Part model, mm, in its own coordinate system. Face numbers are marked on the shaded views. Give positions to 0.01 mm unless a question says otherwise; leave off trailing zeros. Loops run counter-clockwise (first coordinate to the right, second up) from the corner with the lowest first, then second, coordinate; pieces in that order, holes last. Notation, with made-up numbers: (84, -17) -> (102, -17) arc R28 cw to (102, 18) -> close; hole circle Ø9 at (-31, 85). An arc over 180 degrees is marked (long way). One line per question, with ' | ' between items.
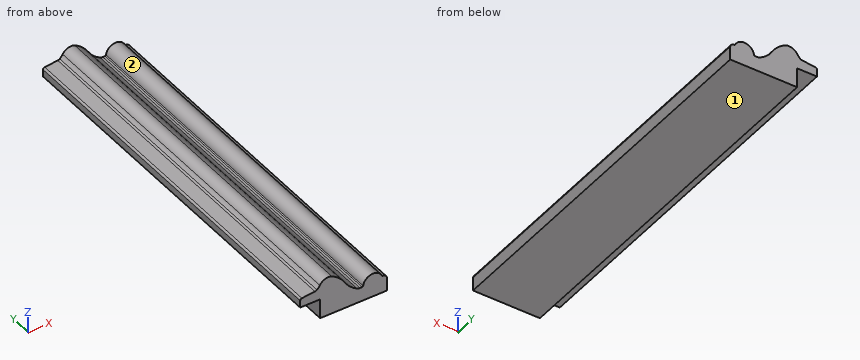
```python
from build123d import *

# Parameters (mm, degrees)
F1_DEPTH = 152.4


# Not quite as in the source:
# - ends of sketch curves that miss each other by under 0.0002 mm in the source are joined


with BuildPart() as f1:
    # F0 (on Front) → F1 (new body)
    with BuildSketch(Plane.XZ):
        with BuildLine():
            Line((-9.4615, 0.028575), (-9.4615, -7.908925))
            Line((-9.4615, -7.908925), (17.4625, -7.908925))
            Line((17.4625, -7.908925), (17.4625, -2.65938))
            ThreePointArc((17.4625, -2.65938), (16.9760741715, -1.5035311682), (15.8095437434, -1.0433101682))
            ThreePointArc((15.8095437434, -1.0433101682), (15.5930919547, -0.9817228233), (15.4491526844, -0.8087322213))
            ThreePointArc((15.4491526844, -0.8087322213), (11.2653307166, 1.5970590296), (7.8607199392, -1.8235935338))
            ThreePointArc((7.8607199392, -1.8235935338), (7.736905149, -2.0587727487), (7.4894692803, -2.1557927219))
            Line((7.4894692803, -2.1557927219), (7.4829161901, -2.1558009151))
            Line((7.4829161901, -2.1558009151), (6.603492, -2.1559774))
            ThreePointArc((6.603492, -2.1559774), (5.9901232061, -2.0809037525), (5.413035163, -1.8599360759))
            ThreePointArc((5.413035163, -1.8599360759), (2.7666336142, 0.0131384296), (0.682874392, 2.4970459891))
            ThreePointArc((0.682874392, 2.4970459891), (-1.6202189431, 5.441919304), (-4.6831053409, 7.585571483))
            ThreePointArc((-4.6831053409, 7.585571483), (-7.435761648, 7.7094554069), (-9.5520790293, 5.9448968563))
            ThreePointArc((-9.5520790293, 5.9448968563), (-10.089729001, 5.2101835463), (-10.7216915696, 4.5548251488))
            ThreePointArc((-10.7216915696, 4.5548251488), (-11.0931160448, 4.3208677831), (-11.52199893, 4.2273251642))
            ThreePointArc((-11.52199893, 4.2273251642), (-14.1558174385, 3.9550500254), (-16.7874935974, 3.6627947922))
            ThreePointArc((-16.7874935974, 3.6627947922), (-17.2692415305, 3.4129116875), (-17.4625, 2.9057854))
            Line((-17.4625, 2.9057854), (-17.4625, 0.028575))
            Line((-17.4625, 0.028575), (-9.4615, 0.028575))
        make_face()
    extrude(amount=F1_DEPTH)


solid = f1.part
```
1) Pin check, flat tips, straight feed: P1, Ø0.7, axis at x = 7, y = -104.5, coming from the +Z side; P2, Ø4, axis at x = 9.5, y = -16.5, coming from the +Z side; P3, Ø6.5, axis at x = -14.5, y = -89, coming from the -Z side. Stop position of each tip, or through.
Found:
P1: z = -2.16 | P2: z = 1.62 | P3: z = 0.03
2) Saw through at C-C (x = -3). Give the cut face in (y, z), and give its area (3 significant figures).
Found:
outline: (-152.4, -7.91) -> (0, -7.91) -> (0, 6.58) -> (-152.4, 6.58) -> close | area: 2,210 mm2
3) Drill centre lines: line 1 (Z direction, x = 15, y = -114.5); line 2 (X direction, y = -98.5, z = -3.25); line 3 (Z direction, x = -6.5, y = -24). Where is each one in solid material? Low to high.
Found:
line 1: -7.91 to -0.01 | line 2: -9.46 to 17.46 | line 3: -7.91 to 7.9
4) Pull direction X, two halves, no side cores. Call the marked faces 1 and 2: pulls with the +X half, pulls with the -X half, needs draft (parallel to the pull), parting line crosses it, or undercut.
Found:
face 1: needs draft | face 2: undercut
5) Saw through at B-B (z = -6.5). Give the cut face in (x, y), and give its area (3 significant figures).
Found:
outline: (-9.46, -152.4) -> (17.46, -152.4) -> (17.46, 0) -> (-9.46, 0) -> close | area: 4,100 mm2
